Read the model definition and answer for the solid it produces. Units are mm, in the model's axes. Face numbers are marked on the shaded views. A direction names the side the tool comes from. Give positions to 0.01 mm unless a question says otherwise; leave off trailing zeros. Write each loop counter-clockwise with the first axis right and the second up, starting at its lowest first coordinate (ties: lowest second). Pieces come first, ordered by that corner, then holes.
```python
from build123d import *
from OCP.BRepFilletAPI import BRepFilletAPI_MakeChamfer

# Parameters (mm, degrees)
BOSS_EXTRUDE3_DEPTH     = 18.796
CUT_EXTRUDE1_START      = -10.414
CUT_EXTRUDE1_DEPTH      = 10.414
CUT_EXTRUDE_THIN1_DEPTH = 4.064
CUT_EXTRUDE2_START      = -3.302
CUT_EXTRUDE2_DEPTH      = 3.302
CHAMFER1_SIZE           = 0.5
CHAMFER1_SIZE2          = 0.491348578


with BuildPart() as part:
    # Sketch2 → Boss-Extrude3 (new body)
    with BuildSketch(Plane(origin=(0, 0, 0), x_dir=(1, 0, 0), z_dir=(0, 1, 0))):
        with BuildLine():
            Line((0, 0), (0, 21.971))
            ThreePointArc((0, 21.971), (15.535843089, 15.535843089), (21.971, 0))
            Line((21.971, 0), (0, 0))
        make_face()
    extrude(amount=BOSS_EXTRUDE3_DEPTH)

    # Sketch4 → Cut-Extrude1 (cut)
    with BuildSketch(Plane(origin=(0, 18.796, 0), x_dir=(1, 0, 0), z_dir=(0, 1, 0)).offset(CUT_EXTRUDE1_START)):
        with BuildLine():
            Line((18.288, 0), (21.971, 0))
            ThreePointArc((21.971, 0), (15.535843089, 15.535843089), (0, 21.971))
            Line((0, 21.971), (0, 18.288))
            ThreePointArc((0, 18.288), (12.931568814, 12.931568814), (18.288, 0))
        make_face()
    extrude(amount=CUT_EXTRUDE1_DEPTH, mode=Mode.SUBTRACT)

    # Sketch5 → Cut-Extrude-Thin1 (cut)
    with BuildSketch(Plane.XZ):
        with BuildLine():
            ThreePointArc((21.971, 0), (15.535843089, -15.535843089), (0, -21.971))
            Line((0, -21.971), (0, -19.431))
            ThreePointArc((0, -19.431), (13.739791865, -13.739791865), (19.431, 0))
            Line((19.431, 0), (21.971, 0))
        make_face()
        with BuildLine():
            ThreePointArc((0, -18.288), (12.931568814, -12.931568814), (18.288, 0))
            Line((18.288, 0), (20.828, 0))
            ThreePointArc((20.828, 0), (14.727620039, -14.727620039), (0, -20.828))
            Line((0, -20.828), (0, -18.288))
        make_face()
    extrude(amount=-CUT_EXTRUDE_THIN1_DEPTH, mode=Mode.SUBTRACT)

    # Sketch6 → Cut-Extrude2 (cut)
    with BuildSketch(Plane(origin=(0, 8.382, 0), x_dir=(1, 0, 0), z_dir=(0, 1, 0)).offset(CUT_EXTRUDE2_START)):
        with BuildLine():
            Line((0, 18.288), (0, 20.574))
            ThreePointArc((0, 20.574), (14.548014916, 14.548014916), (20.574, 0))
            Line((20.574, 0), (18.288, 0))
            ThreePointArc((18.288, 0), (12.931568814, 12.931568814), (0, 18.288))
        make_face()
    extrude(amount=CUT_EXTRUDE2_DEPTH, mode=Mode.SUBTRACT)

    # Chamfer1: one chamfer whose edges measure the first distance from different faces: ONE call of the kernel's chamfer builder (chamfer() names one face for all edges)
    chamfer1_edges_1 = [part.edges().sort_by_distance(p)[0] for p in [
        (15.535843089, 8.382, -15.535843089),
    ]]
    chamfer1_side_1 = [part.faces().sort_by_distance(p)[0] for p in [
        (15.535843089, 6.223, -15.535843089),
    ]]
    chamfer1_edges_2 = [part.edges().sort_by_distance(p)[0] for p in [
        (12.931568814, 18.796, -12.931568814),
    ]]
    chamfer1_side_2 = [part.faces().sort_by_distance(p)[0] for p in [
        (7.761668265, 18.796, -7.761668265),
    ]]
    chamfer1 = BRepFilletAPI_MakeChamfer(part.part.solid().wrapped)
    for e in chamfer1_edges_1:
        chamfer1.Add(CHAMFER1_SIZE, CHAMFER1_SIZE2, e.wrapped, chamfer1_side_1[0].wrapped)  # the first distance lies on this face
    for e in chamfer1_edges_2:
        chamfer1.Add(CHAMFER1_SIZE, CHAMFER1_SIZE2, e.wrapped, chamfer1_side_2[0].wrapped)  # the first distance lies on this face
    add(Compound.cast(chamfer1.Shape()), mode=Mode.REPLACE)


solid = part.part
```
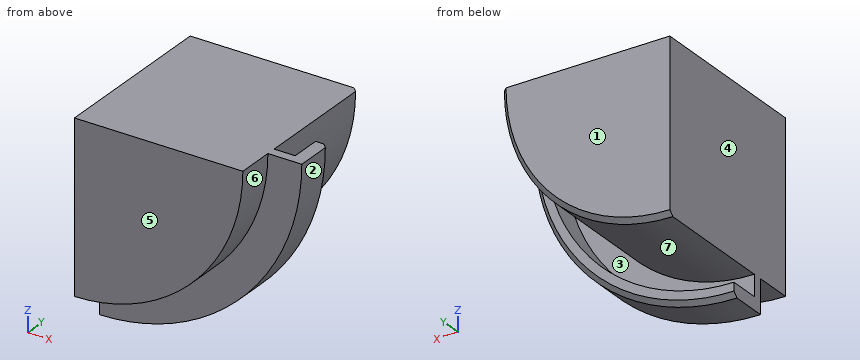
Item 1: Each of these flat-tipped pins is pushed along its axis until it touches: pin 1 Ø10 at (y, z) = (15, -13.5) entering from +X; pin 2 Ø1 at (x, z) = (17, -10) entering from +Y. Where does it stop, or does it pass through?
Result set:
pin 1: stops at x = 16.19
pin 2: stops at y = 5.08
Item 2: Determine the mould class of the marked faces 1, 2, 3 and 4 for opening direction X: pulls with the +X half, pulls with the -X half, needs draft (parallel to the pull), parting line crosses it, or undercut.
Result set:
face 1: needs draft
face 2: pulls with the +X half
face 3: undercut
face 4: pulls with the -X half
Item 3: Section A-A (y = 4.5) is taken. Write down the section's boundary in (x, z), and give its area (3 significant figures).
Result set:
outline: (0, -21.97) arc R21.97 ccw to (21.97, 0) - (0, 0) - close
area: 379 mm2
Item 4: Section B-B (y = 12) is taken. Write down the section's boundary in (x, z).
Result set:
outline: (0, -18.29) arc R18.29 ccw to (18.29, 0) - (0, 0) - close
Item 5: Which of the six approach directions +Z, -Z, +X, -X, +Y, -Y give full straight-line access (tool end or side, diameter ignored) to the marked faces 5, 6 and 7?
Result set:
face 5: +Z, -Z, +X, -X, -Y
face 6: -Z, +X, -Y
face 7: +Y
Item 6: Find the intervals of material crossed by line 1 along Y through (x, z) = (9.75, -16); line 2 along Z through (x, y) = (3.5, 7.75); line 3 along X through (y, z) = (5.5, -16), in increasing order.
Result set:
line 1: y = 4.06 to 5.08
line 2: z = -21.69 to -20.27, -17.95 to 0
line 3: x = 0 to 8.86, 12.93 to 15.06
